from build123d import *

# Parameters (mm, degrees)
SKETCH_21_W    = 1.65
SKETCH_21_H    = 15
CHAMFER_1_SIZE = 0.2


with BuildPart() as part:
    # Эскиз1 → Revolve 921 (revolve)
    with BuildSketch(Plane.XY, mode=Mode.PRIVATE) as revolve_921_sk:
        Polygon((13.75, 9.55), (13.75, 24.25), (15, 25.5), (15, 27), (2.5, 27), (2.5, 2.5), (11.5, 2.5), (11.5, 0), (15, 0), (15, 8.3), align=None)
    revolve(revolve_921_sk.sketch.rotate(Axis((0, 0, 0), (0, 1, 0)), 90), axis=Axis((0, 0, 0), (0, 1, 0)))

    # Эскиз21 → Фиксатор-M4 (revolve, cut)
    with BuildSketch(Plane(origin=(0, 6.25, 0), x_dir=(0, 1, 0), z_dir=(1, 0, 0))):
        with Locations((0.825, 7.5)):
            Rectangle(SKETCH_21_W, SKETCH_21_H)
    revolve(axis=Axis((0, 6.25, -6.35), (0, 0, 1)), mode=Mode.SUBTRACT)

    # Фаска1
    chamfer_1_edges = [part.edges().sort_by_distance(p)[0] for p in [
        (0, 0, 15),
        (0, 0, 11.5),
        (0, 2.5, 2.5),
        (0, 27, 2.5),
        (0, 27, 15),
    ]]
    chamfer(chamfer_1_edges, length=CHAMFER_1_SIZE)


solid = part.part
For this review, take the finished solid that the model builds, in its own axes (mm). A direction names the side the tool comes from. Round coordinates to 2 decimals unless told otherwise and drop trailing zeros. Loops run counter-clockwise (first coordinate to the right, second up) from the corner with the lowest first, then second, coordinate; pieces in that order, holes last. Notation, with made-up numbers: (-36, 86.5) - (11, 86.5) arc R19 ccw to (11, 113.5) - close; hole circle Ø1 at (43, -4.75). An arc over 180 degrees is marked (long way). Use one line per item in the form item = value.
1) Tool access review of faces 4 (the face through (-0.07, 4.6, 8.53)), 5 (the face through (-11.4, 1.3, 1.5)), 6 (the face through (-4.506, 4.307, -14.307)): name each direction out of +Z, -Z, +X, -X, +Y, -Y from which nothing blocks a thin tool from reaching the whole face with its end or side.
Solutions:
face_4 = +Z
face_5 = -Y
face_6 = +Y, -Y
2) Mouldability with a two-part tool opening along Y and no side actions: class faces 1 (the face through (-3, 2.5, 0)), 2 (the face through (-12.65, 26.16, -8.06)), 3 (the face through (12.2, 17, -6.34)) as pulls with the +Y half, pulls with the -Y half, needs draft (parallel to the pull), parting line crosses it, or undercut.
Solutions:
face_1 = pulls with the -Y half
face_2 = needs draft
face_3 = undercut
3) We need section B-B on y = 15. Write out the cut boundary in (x, z).
Solutions:
outline = circle Ø27.5 at (0, 0); hole circle Ø5 at (0, 0)
4) Wall thickness on probe 1 along X at (y, z) = (2, 0); probe 2 along X at (y, z) = (7, 0); probe 3 along Y at (x, z) = (0, 6.75): over which ranges is each line inside the solid? List them lowest first.
Solutions:
probe_1 = -15 to -11.5, 11.5 to 15
probe_2 = -15 to -2.5, 2.5 to 15
probe_3 = 2.5 to 4.6, 7.9 to 27
5) We need section C-C on y = 6.25. Write out the cut boundary in (x, z).
Solutions:
outline = (-1.65, 1.88) - (-1.65, 14.91) arc R15 ccw (long way) to (1.65, 14.91) - (1.65, 1.88) arc R2.5 cw (long way) to start
6) Clearance check with flat-ended pins moving along their axes: P1, Ø6, axis at x = 0, z = 0, coming from the -Y side; P2, Ø1, axis at y = 21, z = -11, coming from the -X side; P3, Ø1.5, axis at x = 10.5, y = 6, coming from the +Z side. State where each tip first meets the part, or that it passes through.
Solutions:
P1 = 2.5
P2 = -8.88
P3 = 11.4
